```python
from build123d import *

# Parameters (mm, degrees)
SKETCH2_R             = 1.778
BOSS_EXTRUDE2_DEPTH   = 16.764
BOSS_EXTRUDE2_2_DEPTH = 16.764
BOSS_EXTRUDE2_3_DEPTH = 16.764
BOSS_EXTRUDE2_4_DEPTH = 16.764
SKETCH2_4_W           = 82.296
SKETCH2_4_H           = 88.392
SKETCH2_4_R           = 1.778
BOSS_EXTRUDE3_DEPTH   = 5.08
SKETCH5_W             = 6.858
SKETCH5_H             = 6.35
BOSS_EXTRUDE4_DEPTH   = 10.16


with BuildPart() as part:
    # Sketch2 → Boss-Extrude2 (new body)
    with BuildSketch(Plane(origin=(0, 0, 0), x_dir=(1, 0, 0), z_dir=(0, 1, 0))):
        with Locations(Location((37.719, -41.021, 0), (0, 0, 270))):
            Circle(SKETCH2_R)
    extrude(amount=BOSS_EXTRUDE2_DEPTH)



with BuildPart() as body_2:
    # Sketch2 → Boss-Extrude2 2 (new body)
    with BuildSketch(Plane(origin=(0, 0, 0), x_dir=(1, 0, 0), z_dir=(0, 1, 0))):
        with Locations(Location((-37.719, -41.021, 0), (0, 0, 90))):
            Circle(SKETCH2_R)
    extrude(amount=BOSS_EXTRUDE2_2_DEPTH)


with BuildPart() as body_3:
    # Sketch2 → Boss-Extrude2 3 (new body)
    with BuildSketch(Plane(origin=(0, 0, 0), x_dir=(1, 0, 0), z_dir=(0, 1, 0))):
        with Locations(Location((37.719, 41.021, 0), (0, 0, 90))):
            Circle(SKETCH2_R)
    extrude(amount=BOSS_EXTRUDE2_3_DEPTH)


with BuildPart() as body_4:
    # Sketch2 → Boss-Extrude2 4 (new body)
    with BuildSketch(Plane(origin=(0, 0, 0), x_dir=(1, 0, 0), z_dir=(0, 1, 0))):
        with Locations(Location((-37.719, 41.021, 0), (0, 0, 270))):
            Circle(SKETCH2_R)
    extrude(amount=BOSS_EXTRUDE2_4_DEPTH)


with BuildPart() as part_1:
    add(part.part)

    add(body_2.part)  # Boss-Extrude3 merges body 2

    add(body_3.part)  # Boss-Extrude3 merges body 3

    add(body_4.part)  # Boss-Extrude3 merges body 4
    # Sketch2_4 → Boss-Extrude3 (add)
    with BuildSketch(Plane(origin=(0, 0, 0), x_dir=(1, 0, 0), z_dir=(0, 1, 0))):
        Rectangle(SKETCH2_4_W, SKETCH2_4_H)
        with Locations(Location((37.719, -41.021, 0), (0, 0, 90))):
            Circle(SKETCH2_4_R, mode=Mode.SUBTRACT)
        with Locations(Location((-37.719, -41.021, 0), (0, 0, 90))):
            Circle(SKETCH2_4_R, mode=Mode.SUBTRACT)
        with Locations(Location((37.719, 41.021, 0), (0, 0, 90))):
            Circle(SKETCH2_4_R, mode=Mode.SUBTRACT)
        with Locations(Location((-37.719, 41.021, 0), (0, 0, 90))):
            Circle(SKETCH2_4_R, mode=Mode.SUBTRACT)
    extrude(amount=BOSS_EXTRUDE3_DEPTH)

    # Sketch5 → Boss-Extrude4 (add)
    with BuildSketch(Plane(origin=(0, 5.08, 0), x_dir=(1, 0, 0), z_dir=(0, 1, 0))):
        with Locations((-37.719, 41.021)):
            Rectangle(SKETCH5_W, SKETCH5_H)
        with Locations((37.719, -41.021)):
            Rectangle(SKETCH5_W, SKETCH5_H)
        with Locations((-37.719, -41.021)):
            Rectangle(SKETCH5_W, SKETCH5_H)
        with Locations((37.719, 41.021)):
            Rectangle(SKETCH5_W, SKETCH5_H)
    extrude(amount=BOSS_EXTRUDE4_DEPTH)


solid = part_1.part
```
CAD build for the part. Positions are in the model's coordinates, mm. A direction names the side the tool comes from. Give positions to 0.01 mm unless a question says otherwise; leave off trailing zeros. Loops run counter-clockwise (first coordinate to the right, second up) from the corner with the lowest first, then second, coordinate; pieces in that order, holes last. Notation, with made-up numbers: M -35,35 L 4,35 A20 cw 4,57 Z; hole C 53,18 d2. An arc over 180 degrees is marked long. Use one line per item in the form item = value.
Item 1: Two-plate mould, pull along X, no slides. Class faces 4 (the face through (-38, 10, -37.846)), 5 (the face through (-34.29, 10, 41)), 6 (the face through (-41.148, 4, 1)), 7 (the face through (41.148, 4, 1)): pulls with the +X half, pulls with the -X half, needs draft (parallel to the pull), parting line crosses it, or undercut.
Determined:
face_4 = needs draft
face_5 = undercut
face_6 = pulls with the -X half
face_7 = pulls with the +X half
Item 2: Slice it at A-A (y = 10.25). List the corners of the cut face in (x, z).
Determined:
outline = M -41.15,-44.2 L -34.29,-44.2 L -34.29,-37.85 L -41.15,-37.85 Z; M -41.15,37.85 L -34.29,37.85 L -34.29,44.2 L -41.15,44.2 Z; M 34.29,-44.2 L 41.15,-44.2 L 41.15,-37.85 L 34.29,-37.85 Z; M 34.29,37.85 L 41.15,37.85 L 41.15,44.2 L 34.29,44.2 Z
Item 3: Slice it at C-C (z = -22.5). List the corners of the cut face in (x, y), plus the area to 3 significant figures.
Determined:
outline = M -41.15,0 L 41.15,0 L 41.15,5.08 L -41.15,5.08 Z
area = 418 mm2
Item 4: Slice it at B-B (x = 27). List the corners of the cut face in (y, z).
Determined:
outline = M 0,-44.2 L 5.08,-44.2 L 5.08,44.2 L 0,44.2 Z
Item 5: Flat gauge pin, fed straight in: pin 1 (3 mm diameter, centred on x = -2.5, z = 28.5, fed in from +Y). Where does the tip first touch, or does it go through?
Determined:
pin_1 = 5.08
Item 6: Drill centre lines: probe 1 along Y at (x, z) = (-36.5, 30.5); probe 2 along Z at (x, y) = (38, 8.5). Where is each one in solid material? Low to high. Write a range as from..to.
Determined:
probe_1 = 0..5.08
probe_2 = -44.2..-37.85, 37.85..44.2
Item 7: Which spindle directions (+Z, -Z, +X, -X, +Y, -Y) get a long thin tool onto all of the face, cutting with end or side? Do faces 1 (the face through (38, 10, 37.846)), 2 (the face through (34.29, 10, -41)), 3 (the face through (37.641, 15.991, -39.245)). Say none if no direction does.
Determined:
face_1 = +X, -X, +Y
face_2 = +Z, -Z, +Y
face_3 = +Y
